Read the model definition and answer for the solid it produces. Units are mm, in the model's axes. Give positions to 0.01 mm unless a question says otherwise; leave off trailing zeros. Loops run counter-clockwise (first coordinate to the right, second up) from the corner with the lowest first, then second, coordinate; pieces in that order, holes last. Notation, with made-up numbers: M -34.75,-28 L -11.75,-28 A24 ccw -11.75,7 Z; hole C 81.5,77 d5. An arc over 180 degrees is marked long. Return JSON: item names as keys, results as strings. Group by question number.
```python
from build123d import *

# Parameters (mm, degrees)
SKETCH_1_R          = 21.5
SKETCH_1_R_2        = 18
EXTRUDE_1_DEPTH     = 5
SKETCH_2_R          = 10.025
CUT_EXTRUDE_1_DEPTH = 31.813957876
SKETCH_3_R          = 2.05
CUT_EXTRUDE_2_DEPTH = 31.813957876


with BuildPart() as part:
    # ｽｹｯﾁ1 → ﾎﾞｽ - 押し出し1 (new body)
    with BuildSketch(Plane.XY):
        Circle(SKETCH_1_R)
        Circle(SKETCH_1_R_2, mode=Mode.SUBTRACT)
        Circle(SKETCH_1_R_2)
    extrude(amount=EXTRUDE_1_DEPTH)

    # ｽｹｯﾁ2 → ｶｯﾄ - 押し出し1 (cut, through all)
    with BuildSketch(Plane.XY.offset(5)):
        Circle(SKETCH_2_R)
    extrude(amount=-CUT_EXTRUDE_1_DEPTH, mode=Mode.SUBTRACT)

    # ｽｹｯﾁ3 → ｶｯﾄ - 押し出し2 (cut, through all)
    with BuildSketch(Plane.XY.offset(5)):
        with Locations((0, -17)):
            Circle(SKETCH_3_R)
        with Locations((-14.722431864, 8.5)):
            Circle(SKETCH_3_R)
        with Locations((14.722431864, 8.5)):
            Circle(SKETCH_3_R)
    extrude(amount=-CUT_EXTRUDE_2_DEPTH, mode=Mode.SUBTRACT)


solid = part.part
```
1. Find section A-A (y = 0). Write down the section's boundary in (x, z) (3 decimals).
2. The mould has two halves that part along Y. Classify faces 1 (the flat face through (4.5, -9.3, 5)), 2 (the cylindrical face through (-2.799, 21.317, 2.465)), 3 (the cylindrical face through (16.616, 7.715, 2.535)): +Y half, -Y half, draft (parallel to the pull), parting line (faces both ways), or undercut.
3. Flat-ended cylindrical pins translate along their axes: P1, Ø2, axis at y = 11.5, z = 1, coming from the +X side; P2, Ø1.5, axis at x = 0, z = 2.5, coming from the +Y side; P3, Ø1.5, axis at y = 13, z = 2.5, coming from the -X side. Find the tip coordinate at first contact, or state that the pin passes through.
4. Find section C-C (x = -15). Write down the section's boundary in (y, z).
5. Straight lines are drawn through the part: line 1 along Y through (x, z) = (0, 1) (3 decimals); line 2 along Y through (x, z) = (-15.5, 1.15); line 3 along X through (y, z) = (-1.5, 1.3). For each, find the intervals that lie inside material, in ascending order.
6. Find section D-D (z = 3.7). Write down the section's boundary in (x, y) (3 decimals), and give its area (3 significant figures).
7. Find section B-B (x = 0). Write down the section's boundary in (y, z) (3 decimals).
Result:
{
 "1": {"outline": "M -21.5,0 L -10.025,0 L -10.025,5 L -21.5,5 Z; M 10.025,0 L 21.5,0 L 21.5,5 L 10.025,5 Z"},
 "2": {"face 1": "draft", "face 2": "parting line", "face 3": "undercut"},
 "3": {"P1": "stops at x = 18.76", "P2": "stops at y = 21.5", "P3": "stops at x = -17.67"},
 "4": {"outline": "M -15.4,0 L 6.47,0 L 6.47,5 L -15.4,5 Z; M 10.53,0 L 15.4,0 L 15.4,5 L 10.53,5 Z"},
 "5": {"line 1": "y = -21.5 to -19.05, -14.95 to -10.025, 10.025 to 21.5", "line 2": "y = -14.9 to 6.6, 10.4 to 14.9", "line 3": "x = -21.45 to -9.91, 9.91 to 21.45"},
 "6": {"outline": "C 0,0 d43; hole C -14.722,8.5 d4.1; hole C 0,0 d20.05; hole C 0,-17 d4.1; hole C 14.722,8.5 d4.1", "area": "1,100 mm2"},
 "7": {"outline": "M -21.5,0 L -19.05,0 L -19.05,5 L -21.5,5 Z; M -14.95,0 L -10.025,0 L -10.025,5 L -14.95,5 Z; M 10.025,0 L 21.5,0 L 21.5,5 L 10.025,5 Z"}
}
